Here's the drawing with two shaded views (mm, measured from the low corner). I have some questions. A direction names the side the tool comes from. Round coordinates to 2 decimals unless told otherwise and drop trailing zeros. Loops run counter-clockwise (first coordinate to the right, second up) from the corner with the lowest first, then second, coordinate; pieces in that order, holes last.
(1) I want a section at C-C on y = 1.5. Write out the boundary of the cut face in (x, z).
(2) If I drill on line 1 along Z through (x, y) = (26.5, 13) (1 decimal); line 2 along X through (y, z) = (11.75, 20); line 3 along Y through (x, z) = (30, 16.5), over which ranges is the centre line in solid material (lowest first)?
(3) I want a section at D-D on z = 61. Write out the boundary of the cut face in (x, y), plus the area to 3 significant figures.
(4) Which directions (+Z, -Z, +X, -X, +Y, -Y) give clear straight access to the entire face, cutting with the end or side of a thin tool? Please do the marked faces 1 and 2.
(5) I want a section at A-A on z = 50.8. Write out the boundary of the cut face in (x, y).
(6) Will these pins go through, and if not, where does the flat tip stop? pin 1 Ø4 at (y, z) = (14.5, 31) entering from -X; pin 2 Ø10 at (x, z) = (9.5, 43.5) entering from +Y; pin 3 Ø5 at (x, y) = (29.5, 15.5) entering from -Z (1 decimal).
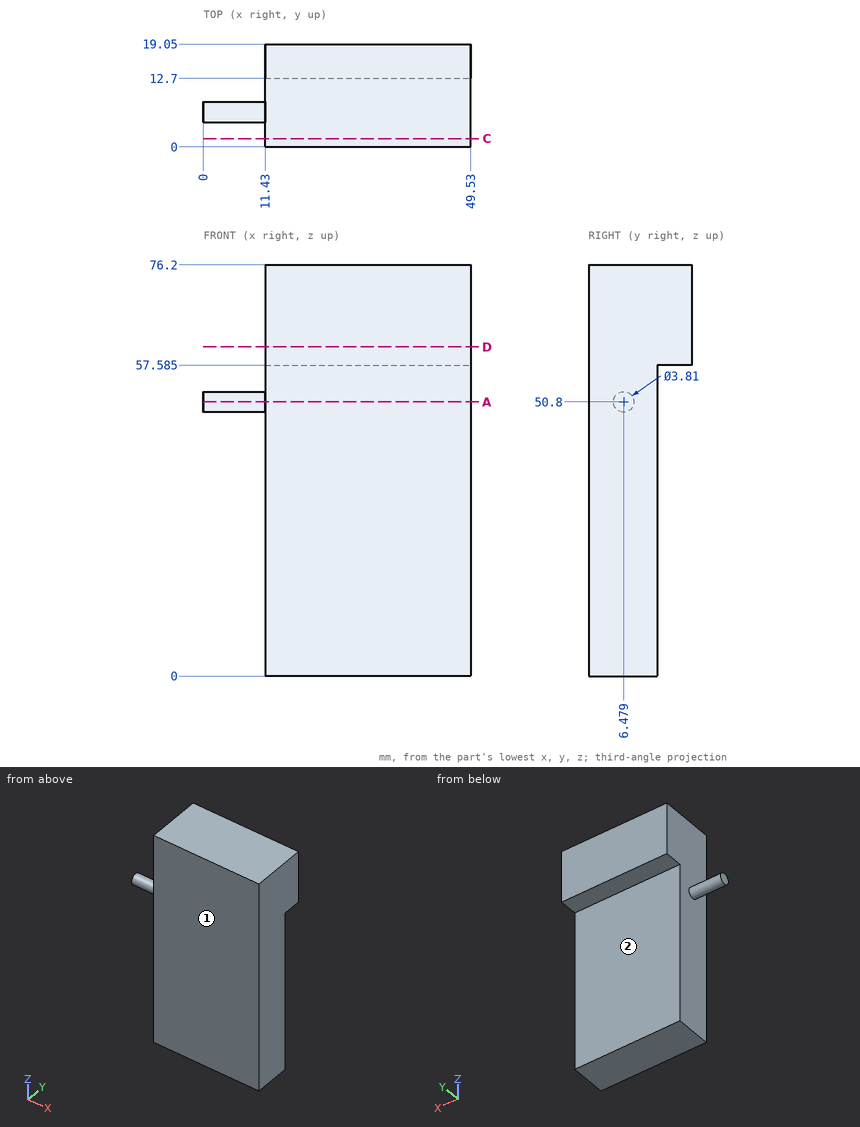
Filled sheet:
1. outline: (11.43, 0) - (49.53, 0) - (49.53, 76.2) - (11.43, 76.2) - close
2. line 1: z = 57.6 to 76.2
2. line 2: x = 11.43 to 49.53
2. line 3: y = 0 to 12.7
3. outline: (11.43, 0) - (49.53, 0) - (49.53, 19.05) - (11.43, 19.05) - close
3. area: 726 mm2
4. face 1: +Z, -Z, +X, -X, -Y
4. face 2: -Z, +X, -X, +Y
5. outline: (0, 4.57) - (11.43, 4.57) - (11.43, 0) - (49.53, 0) - (49.53, 12.7) - (11.43, 12.7) - (11.43, 8.38) - (0, 8.38) - close
6. pin 1: stops at x = 11.43
6. pin 2: stops at y = 12.7
6. pin 3: stops at z = 57.6
